Could you check a few things on this model? Use its own coordinates, in mm. Give positions to 0.01 mm unless a question says otherwise; leave off trailing zeros. Write each loop counter-clockwise with the first axis right and the second up, starting at its lowest first coordinate (ties: lowest second). Pieces come first, ordered by that corner, then holes. Notation, with made-up numbers: (-10.5, 62.25) - (15.5, 62.25) arc R12 ccw to (15.5, 71.25) - close; hole circle Ø8 at (33, 69). An arc over 180 degrees is marked (long way). Answer as a JSON object with one key per item and string values. Group by question number.
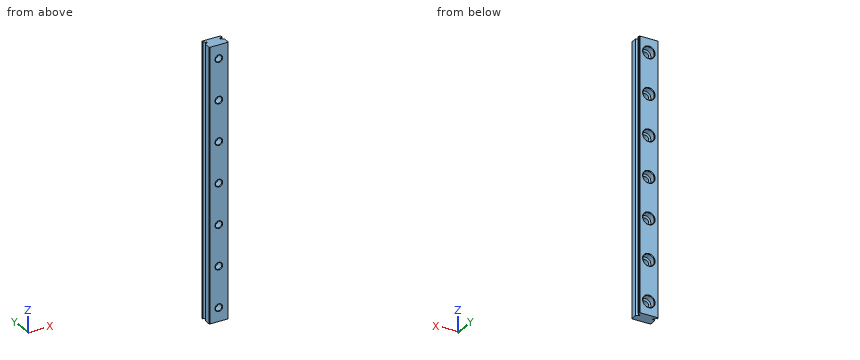
```python
from build123d import *

# Parameters (mm, degrees)
EXTRUDE1_DEPTH             = 100
SKETCH2_R                  = 1.2
EXTRUDE2_DEPTH             = 4.8
SKETCH_R                   = 2.1
SKETCH_R_2                 = 1.2
EXTRUDE4_DEPTH             = 2.3
CHAMFER1_SIZE              = 0.2
LPATTERN1_COUNT            = 7
LPATTERN1_PITCH            = 15
CHAMFER1_OF_LPATTERN1_SIZE = 0.2


with BuildPart() as part:
    # Sketch1 → Extrude1 (new body)
    with BuildSketch(Plane.XY):
        with BuildLine():
            Line((-3.3, -2.4), (3.3, -2.4))
            Line((3.3, -2.4), (3.5, -2.2))
            Line((3.5, -2.2), (3.5, 0.106274607))
            ThreePointArc((3.5, 0.106274607), (3.091294745, 0.282570681), (2.840065792, 0.65))
            Line((2.840065792, 0.65), (2.340065792, 0.65))
            Line((2.340065792, 0.65), (2.340065792, 1.15))
            Line((2.340065792, 1.15), (2.840065792, 1.15))
            ThreePointArc((2.840065792, 1.15), (3.091294745, 1.517429319), (3.5, 1.693725393))
            Line((3.5, 1.693725393), (3.5, 2.2))
            Line((3.5, 2.2), (3.3, 2.4))
            Line((3.3, 2.4), (-3.3, 2.4))
            Line((-3.3, 2.4), (-3.5, 2.2))
            Line((-3.5, 2.2), (-3.5, 1.693725393))
            ThreePointArc((-3.5, 1.693725393), (-3.091294745, 1.517429319), (-2.840065792, 1.15))
            Line((-2.840065792, 1.15), (-2.340065792, 1.15))
            Line((-2.340065792, 1.15), (-2.340065792, 0.65))
            Line((-2.340065792, 0.65), (-2.840065792, 0.65))
            ThreePointArc((-2.840065792, 0.65), (-3.091294745, 0.282570681), (-3.5, 0.106274607))
            Line((-3.5, 0.106274607), (-3.5, -2.2))
            Line((-3.5, -2.2), (-3.3, -2.4))
        make_face()
    extrude(amount=EXTRUDE1_DEPTH)

    # Sketch2 → Extrude2 (cut)
    with BuildSketch(Plane(origin=(0, 2.4, 0), x_dir=(1, 0, 0), z_dir=(0, 1, 0))):
        with Locations((0, -5)):
            Circle(SKETCH2_R)
    extrude2 = extrude(amount=-EXTRUDE2_DEPTH, mode=Mode.SUBTRACT)

    # Sketch → Extrude4 (cut)
    with BuildSketch(Plane(origin=(0, 2.4, 0), x_dir=(1, 0, 0), z_dir=(0, 1, 0))):
        with Locations((0, -5)):
            Circle(SKETCH_R)
        with Locations((0, -5)):
            Circle(SKETCH_R_2, mode=Mode.SUBTRACT)
    extrude4 = extrude(amount=-EXTRUDE4_DEPTH, mode=Mode.SUBTRACT)

    # Chamfer1
    chamfer1_edges = [part.edges().sort_by_distance(p)[0] for p in [
        (-1.2, -2.4, 5),
        (-2.1, 2.4, 5),
    ]]
    chamfer(chamfer1_edges, length=CHAMFER1_SIZE)

    # LPattern1: Extrude2, Extrude4 ×7
    with Locations(*[(0, 0, i * LPATTERN1_PITCH) for i in range(1, LPATTERN1_COUNT)]):
        add(extrude2, mode=Mode.SUBTRACT)
        add(extrude4, mode=Mode.SUBTRACT)

    # Chamfer1 of LPattern1
    chamfer1_of_lpattern1_edges = [part.edges().sort_by_distance(p)[0] for p in [
        (-1.2, -2.4, 20),
        (-2.1, 2.4, 20),
        (-1.2, -2.4, 35),
        (-2.1, 2.4, 35),
        (-1.2, -2.4, 50),
        (-2.1, 2.4, 50),
        (-1.2, -2.4, 65),
        (-2.1, 2.4, 65),
        (-1.2, -2.4, 80),
        (-2.1, 2.4, 80),
        (-1.2, -2.4, 95),
        (-2.1, 2.4, 95),
    ]]
    chamfer(chamfer1_of_lpattern1_edges, length=CHAMFER1_OF_LPATTERN1_SIZE)


solid = part.part
```
(1) I want a section at C-C, the plane z = 89. Please give me the cut outline in (x, y), and give its area (3 significant figures).
(2) I need wall thicknesses on L1, parallel to Y at x = 2.5, z = 92; L2, parallel to X at y = 1, z = 80; L3, parallel to Y at x = -1.5, z = 19. Which ranges of each line are inside material? Lowest first, please.
(3) I want a section at B-B, the plane y = -1.4. Please give me the cut outline in (x, z).
(4) Will these pins go through, and if not, where does the flat tip stop? P1, Ø0.5, axis at y = 1, z = 66.5, coming from the -X side; P2, Ø1.3, axis at x = 0.5, z = 81, coming from the +Y side; P3, Ø2.5, axis at x = 0, z = 20, coming from the -Y side.
Entries:
{
 "1": {"outline": "(-3.5, -2.2) - (-3.3, -2.4) - (3.3, -2.4) - (3.5, -2.2) - (3.5, 0.11) arc R0.8 cw to (2.84, 0.65) - (2.34, 0.65) - (2.34, 1.15) - (2.84, 1.15) arc R0.8 cw to (3.5, 1.69) - (3.5, 2.2) - (3.3, 2.4) - (-3.3, 2.4) - (-3.5, 2.2) - (-3.5, 1.69) arc R0.8 cw to (-2.84, 1.15) - (-2.34, 1.15) - (-2.34, 0.65) - (-2.84, 0.65) arc R0.8 cw to (-3.5, 0.11) - close", "area": "31.4 mm^2"},
 "2": {"L1": "-2.4 to 0.65, 1.15 to 2.4", "L2": "-2.34 to -2.1, 2.1 to 2.34", "L3": "-2.4 to 0.1"},
 "3": {"outline": "(-3.5, 0) - (3.5, 0) - (3.5, 100) - (-3.5, 100) - close; hole circle Ø2.4 at (0, 5); hole circle Ø2.4 at (0, 20); hole circle Ø2.4 at (0, 35); hole circle Ø2.4 at (0, 50); hole circle Ø2.4 at (0, 65); hole circle Ø2.4 at (0, 80); hole circle Ø2.4 at (0, 95)"},
 "4": {"P1": "x = -2.88", "P2": "y = 0.1", "P3": "y = -2.25"}
}
